Build history of the part. All positions in model axes, mm. A direction names the side the tool comes from. Round coordinates to 2 decimals unless told otherwise and drop trailing zeros. Write each loop counter-clockwise with the first axis right and the second up, starting at its lowest first coordinate (ties: lowest second). Pieces come first, ordered by that corner, then holes.
Item 1: Band-saw the part on A-A, the plane z = 306.5. Write the cut outline in (x, y).
Item 2: Drop flat-ended pins along their axis: pin 1 Ø2 at (x, z) = (-6, 199.5) entering from +Y; pin 2 Ø6.5 at (x, z) = (0, 6) entering from +Y; pin 3 Ø4 at (x, y) = (0, 3.5) entering from -Z. Give the stop position or say it passes through.
Item 3: Wall check: probe 1 along Z at (x, y) = (0, -4.25); probe 2 along Z at (x, y) = (-0.25, -7.5); probe 3 along Y at (x, z) = (0, 977.5). Give the ranges that are in metal, low to high.
Item 4: 3-axis set-ups, long thin cutter, end or side, ignore diameter. For faces 1 (the cylindrical face through (-1.172, 8.923, 493)), 2 (the flat face through (0, 1, 13)): which of +Z, -Z, +X, -X, +Y, -Y reach the whole face in a straight line?
```python
from build123d import *

# Parameters (mm, degrees)
CROQUIS1_R              = 9
SALIENTE_EXTRUIR1_DEPTH = 1000
CROQUIS2_R              = 5
CORTAR_EXTRUIR1_DEPTH   = 30
CORTAR_EXTRUIR2_DEPTH   = 26
CROQUIS5_R              = 2.5
CORTAR_EXTRUIR3_DEPTH   = 10


with BuildPart() as part:
    # Croquis1 → Saliente-Extruir1 (new body)
    with BuildSketch(Plane.XY):
        Circle(CROQUIS1_R)
    extrude(amount=SALIENTE_EXTRUIR1_DEPTH)

    # Croquis2 → Cortar-Extruir1 (cut)
    with BuildSketch(Plane.XY.offset(1000)):
        Circle(CROQUIS2_R)
    extrude(amount=-CORTAR_EXTRUIR1_DEPTH, mode=Mode.SUBTRACT)

    # Croquis4 → Cortar-Extruir2 (cut)
    with BuildSketch(Plane(origin=(0, 0, 0), x_dir=(-1, 0, 0), z_dir=(0, 0, -1))):
        with BuildLine():
            Line((-8.94427191, 1), (8.94427191, 1))
            ThreePointArc((8.94427191, 1), (6, 6.708203932), (0, 9))
            ThreePointArc((0, 9), (-6, 6.708203932), (-8.94427191, 1))
        make_face()
    extrude(amount=-CORTAR_EXTRUIR2_DEPTH, mode=Mode.SUBTRACT)

    # Croquis5 → Cortar-Extruir3 (cut)
    with BuildSketch(Plane(origin=(0, 1, 0), x_dir=(1, 0, 0), z_dir=(0, 1, 0))):
        with Locations((0, -6)):
            Circle(CROQUIS5_R)
        with Locations((0, -16)):
            Circle(CROQUIS5_R)
    extrude(amount=-CORTAR_EXTRUIR3_DEPTH, mode=Mode.SUBTRACT)


solid = part.part
```
Results:
1. outline: circle Ø18 at (0, 0)
2. pin 1: stops at y = 7.48
2. pin 2: stops at y = 1
2. pin 3: stops at z = 26
3. probe 1: z = 0 to 3.5, 8.5 to 13.5, 18.5 to 970
3. probe 2: z = 0 to 3.51, 8.49 to 13.51, 18.49 to 1000
3. probe 3: y = -9 to -5, 5 to 9
4. face 1: +Z, -Z
4. face 2: -Z, +X, -X, +Y
